from build123d import *

# Parameters (mm, degrees)
SKETCH1_W = 8.509
SKETCH1_H = 12.7
FILLET2_R = 0.254


with BuildPart() as part:
    # Sketch1 → Revolve1 (revolve)
    with BuildSketch(Plane.XY, mode=Mode.PRIVATE) as revolve1_sk:
        Polygon((0, 0), (2.159, 0), (2.159, 16.002), (0, 16.002), (0, 12.7), align=None)
        with Locations((-4.2545, 6.35)):
            Rectangle(SKETCH1_W, SKETCH1_H)
    revolve(revolve1_sk.sketch.rotate(Axis((6.35, 0, 0), (0, 1, 0)), 270), axis=Axis((6.35, 0, 0), (0, 1, 0)))

    # Fillet2
    fillet2_edges = [part.edges().sort_by_distance(p)[0] for p in [
        (6.35, 0, 14.859),
        (6.35, 12.7, 14.859),
        (6.35, 12.7, 6.35),
        (6.35, 16.002, 6.35),
    ]]
    fillet(fillet2_edges, radius=FILLET2_R)


solid = part.part
For this review, take the finished solid that the model builds, in its own axes (mm). A direction names the side the tool comes from. Round coordinates to 2 decimals unless told otherwise and drop trailing zeros. Write each loop counter-clockwise with the first axis right and the second up, starting at its lowest first coordinate (ties: lowest second). Pieces come first, ordered by that corner, then holes. Notation, with made-up numbers: M 20,32 L 54,32 A15 cw 54,38 Z; hole C 28.25,4.25 d10. An arc over 180 degrees is marked long. Write item = value, one per line. Start each with the question number.
(1) For line 1 along X through (y, z) = (4.75, 0); line 2 along Y through (x, z) = (3.25, -7); line 3 along X through (y, z) = (9, -3.5), list the stretches that pass through material, from the lowest coordinate up.
(2) Clearance check with flat-ended pins moving along their axes: pin 1 Ø1.5 at (x, z) = (2, -8) entering from -Y; pin 2 Ø7.5 at (x, z) = (6.35, 0) entering from -Y; pin 3 Ø1.5 at (x, y) = (10.5, 8) entering from -Z; pin 4 Ø10 at (x, z) = (17, -10.5) entering from +Y. State where each tip first meets the part, or that it passes through.
(3) For faces 4 (the face through (2, 16.002, 1)), 5 (the face through (9.4, 12.7, -6.3)), list the 3-axis set-ups (+Z, -Z, +X, -X, +Y, -Y) from which the entire face can be reached by the end or side of a thin tool; tool diameter is ignored.
(4) We need section B-B (x = 6.35). Give the boundary of the cut face in (y, z) (3 decimals).
(5) The part is to be moulded in two halves that separate along X. For faces 1 (the face through (12.55, 14.33, 1.38)), 2 (the face through (9.4, 0, 3.5)), 3 (the face through (10.44, 8.11, 0.91)), say which applies: +X half, -X half, draft (parallel to the pull), parting line (faces both ways), or undercut.
(6) We need section A-A (z = 0). Give the boundary of the cut face in (x, y) (3 decimals).
(7) We need section C-C (y = 8). Give the boundary of the cut face in (x, z), then the cut area to 3 significant figures.
Results found:
q1.line_1 = -8.51 to 2.16, 10.54 to 21.21
q1.line_2 = 0 to 12.7
q1.line_3 = -8.09 to 4.04, 8.66 to 20.79
q2.pin_1 = 0
q2.pin_2 = through
q2.pin_3 = -14.46
q2.pin_4 = 12.7
q3.face_4 = +Z, -Z, +X, -X, +Y
q3.face_5 = +Y
q4.outline = M 0,-14.605 A0.254 ccw 0.254,-14.859 L 12.446,-14.859 A0.254 ccw 12.7,-14.605 L 12.7,-6.604 A0.254 cw 12.954,-6.35 L 15.748,-6.35 A0.254 ccw 16.002,-6.096 L 16.002,-4.191 L 0,-4.191 Z; M 0,4.191 L 16.002,4.191 L 16.002,6.096 A0.254 ccw 15.748,6.35 L 12.954,6.35 A0.254 cw 12.7,6.604 L 12.7,14.605 A0.254 ccw 12.446,14.859 L 0.254,14.859 A0.254 ccw 0,14.605 Z
q5.face_1 = parting line
q5.face_2 = draft
q5.face_3 = undercut
q6.outline = M -8.509,0.254 A0.254 ccw -8.255,0 L 2.159,0 L 2.159,16.002 L 0.254,16.002 A0.254 ccw 0,15.748 L 0,12.954 A0.254 cw -0.254,12.7 L -8.255,12.7 A0.254 ccw -8.509,12.446 Z; M 10.541,0 L 20.955,0 A0.254 ccw 21.209,0.254 L 21.209,12.446 A0.254 ccw 20.955,12.7 L 12.954,12.7 A0.254 cw 12.7,12.954 L 12.7,15.748 A0.254 ccw 12.446,16.002 L 10.541,16.002 Z
q7.outline = C 6.35,0 d29.72; hole C 6.35,0 d8.38
q7.area = 638 mm²
